CAD build for the part. Positions are in the model's coordinates, mm. Face numbers are marked on the shaded views. A direction names the side the tool comes from. Give positions to 0.01 mm unless a question says otherwise; leave off trailing zeros. Loops run counter-clockwise (first coordinate to the right, second up) from the corner with the lowest first, then second, coordinate; pieces in that order, holes last.
Item 1: Probe probe 1 along Z at (x, y) = (-4.5, -0.5); probe 2 along Z at (x, y) = (-35, -2.5); probe 3 along X at (y, z) = (-6.25, 13). List the from-to ranges inside material, lowest first.
Item 2: Drop flat-ended pins along their axis: P1, Ø5, axis at x = -4.5, y = -1.5, coming from the +Z side; P2, Ø20, axis at x = -10, z = 14, coming from the +Y side; P3, Ø5, axis at x = -19.5, z = 12, coming from the +Y side; P4, Ø8, axis at y = -4, z = 6.5, coming from the -X side. Give the stop position or say it passes through.
Item 3: Saw through at B-B on y = 0. Give the cut face in (x, z), plus the area to 3 significant figures.
Item 4: Saw through at C-C on z = 12. Give the cut face in (x, y).
Item 5: Which spindle directions (+Z, -Z, +X, -X, +Y, -Y) get a long thin tool onto all of the face, cutting with end or side? Do the marked faces 1 and 2. Say none if no direction does.
Item 6: Saw through at A-A on x = -7. Give the cut face in (y, z).
Item 7: Saw through at D-D on y = 5. Give the cut face in (x, z).
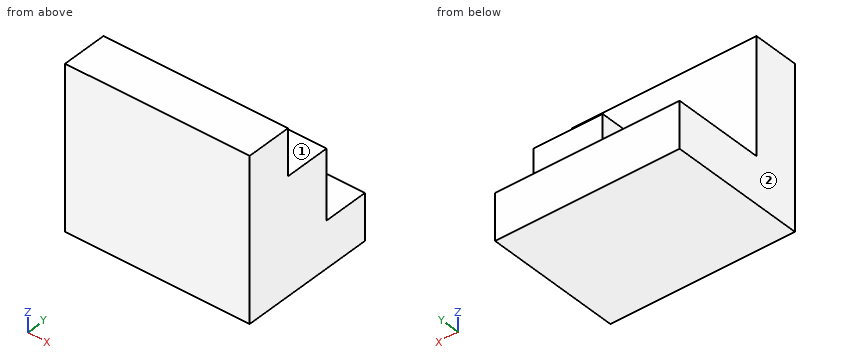
from build123d import *

# Parameters (mm, degrees)
BOSS_EXTRUDE1_DEPTH = 40
SKETCH2_W           = 15
SKETCH2_H           = 10
BOSS_EXTRUDE2_DEPTH = 15


with BuildPart() as part:
    # Sketch1 → Boss-Extrude1 (new body)
    with BuildSketch(Plane(origin=(0, 0, 0), x_dir=(0, 0, -1), z_dir=(1, 0, 0))):
        Polygon((10.105951264, 12.773109244), (10.105951264, -17.226890756), (-24.894048736, -17.226890756), (-24.894048736, -7.226890756), (0.105951264, -7.226890756), (0.105951264, 12.773109244), align=None)
    extrude(amount=-BOSS_EXTRUDE1_DEPTH)

    # Sketch2 → Boss-Extrude2 (add)
    with BuildSketch(Plane(origin=(0, 0, 0), x_dir=(0, 0, -1), z_dir=(1, 0, 0))):
        with Locations((-7.394048736, -2.226890756)):
            Rectangle(SKETCH2_W, SKETCH2_H)
    extrude(amount=-BOSS_EXTRUDE2_DEPTH)


solid = part.part
Results below:
1. probe 1: z = -10.11 to 14.89
1. probe 2: z = -10.11 to -0.11
1. probe 3: x = -15 to 0
2. P1: stops at z = 14.89
2. P2: stops at y = 2.77
2. P3: stops at y = -7.23
2. P4: stops at x = -40
3. outline: (-40, -10.11) - (0, -10.11) - (0, 14.89) - (-15, 14.89) - (-15, -0.11) - (-40, -0.11) - close
3. area: 625 mm2
4. outline: (-40, -17.23) - (0, -17.23) - (0, 2.77) - (-15, 2.77) - (-15, -7.23) - (-40, -7.23) - close
5. face 1: +Z, +X, -X, +Y
5. face 2: +Z, -Z, -X, +Y, -Y
6. outline: (-17.23, -10.11) - (12.77, -10.11) - (12.77, -0.11) - (2.77, -0.11) - (2.77, 14.89) - (-7.23, 14.89) - (-7.23, 24.89) - (-17.23, 24.89) - close
7. outline: (-40, -10.11) - (0, -10.11) - (0, -0.11) - (-40, -0.11) - close
